Autodesk Inventor part; units mm, degrees
ref_plane "YZ Plane" through (0, 0, 0) normal (1, 0, 0) x (0, 1, 0)
ref_plane "XZ Plane" through (0, 0, 0) normal (0, 1, 0) x (-1, 0, 0)
ref_plane "XY Plane" through (0, 0, 0) normal (0, 0, 1) x (1, 0, 0)
sketch "Sketch1" plane through (0, 0, 0) normal (0, 1, 0) x (-1, 0, 0)
  line L0 (-15, 20.25) -> (15, 20.25)
  line L1 (15, 20.25) -> (15, -20.25)
  line L2 (15, -20.25) -> (-15, -20.25)
  line L3 (-15, -20.25) -> (-15, 20.25)
  line L4 (-15, 20.25) -> (15, -20.25) construction
  line L5 (15, 20.25) -> (-15, -20.25) construction
  point P0 (0, 0)
  dimension "d0" = 40.5
  dimension "d1" = 30
extrude "Plate1" add sketch "Sketch1" along normal blind 1.5
sketch "Sketch2" plane through (-15, 0, -21.75) normal (0, 0, 1) x (1, 0, 0)
  line L0 (30, 0) -> (0, 0)
  line L1 (0, 0) -> (0, 33.4)
  line L2 (0, 33.4) -> (30, 33.4)
  line L3 (30, 33.4) -> (30, 0)
edge flange "Flange1" height 33.4 angle 90 thickness 1.5 bend radius 0.31 thickness toward (0, 0, 1) relief tear relief width 1.5 relief depth 0.75 corner gap 0.31 corner form 0 edges at (0, 1.5, -20.25) (0, 1.5, 20.25) wall of the first edge with corners at (15, 0, -21.75) (-15, 0, -21.75) (-15, 33.4, -21.75) (15, 33.4, -21.75)
bend "Bend1"
corner "Corner1"
sketch "Sketch3" plane through (0, 1.5, 0) normal (0, 1, 0) x (1, 0, 0)
  circle A0 centre (7, 0) radius 0.7835
  circle A1 centre (0, -7) radius 0.7835
  circle A2 centre (-7, 0) radius 0.7835
  circle A3 centre (0, 7) radius 0.7835
  point P0 (0, 0)
hole "Hole1" at (0, 1.5, 7) at (7, 1.5, 0) at (-7, 1.5, 0) at (0, 1.5, -7) direction (0, -1, 0) diameter 2.1 depth 1.5
sketch "Sketch26" plane through (-15, 33.4, 21.75) normal (0, 0, 1) x (1, 0, 0)
  line L0 (30, 11.6) -> (25, 11.6)
  line L1 (25, 11.6) -> (25, -23.4)
  line L2 (25, -23.4) -> (30, -23.4)
  line L3 (30, -23.4) -> (30, 11.6)
  line L4 (0, 11.6) -> (5, 11.6)
  line L5 (5, 11.6) -> (5, -23.4)
  line L6 (5, -23.4) -> (0, -23.4)
  line L7 (0, -23.4) -> (0, 11.6)
  point P0 (15, -33.4)
  dimension "d91" = 35
  dimension "d92" = 5
  dimension "d93" = 10
  dimension "d94" = 10
  dimension "d95" = 5
  dimension "d96" = 35
  dimension "d97" = 10
  dimension "d98" = 10
extrude "Cut11" cut sketch "Sketch26" against normal blind 1.5
fillet "Corner Round1" radius 5 1 edges at (-15, 10, 21)
fillet "Corner Round2" radius 5 1 edges at (15, 10, 21)
mirror "Mirror1" about plane through (0, 0, 0) normal (0, 0, 1) of "Cut11"
fillet "Corner Round3" radius 5 1 edges at (-15, 10, -21)
fillet "Corner Round4" radius 5 1 edges at (15, 10, -21)
sketch "Sketch27" plane through (-15, 1.81, 21.75) normal (0, 0, 1) x (1, 0, 0)
  circle A0 centre (15, 32.29) radius 6
  point P0 (15, -1.81)
extrude "Cut12" cut sketch "Sketch27" against normal blind 1.5
sketch "Sketch28" plane through (15, 1.81, -21.75) normal (0, 0, -1) x (-1, 0, 0)
  circle A0 centre (15, 32.29) radius 6
  point P0 (15, -1.81)
extrude "Cut13" cut sketch "Sketch28" against normal blind 1.5
fillet "Corner Round5" radius 1 4 edges at (10, 33.4, -21) (10, 33.4, 21) (-10, 33.4, 21) (-10, 33.4, -21)
sketch "Sketch31" plane through (-15, 1.81, 21.75) normal (0, 0, 1) x (1, 0, 0)
  point P0 (15, -1.81)
sketch "Sketch32" plane through (-15, 1.81, 21.75) normal (0, 0, 1) x (1, 0, 0)
  circle A0 centre (23, 25.39) radius 0.7835
  circle A1 centre (22, 12.17) radius 0.7835
  circle A2 centre (7, 25.39) radius 0.7835
  circle A3 centre (8, 12.17) radius 0.7835
  circle A4 centre (15, 4.87) radius 0.7835
  point P0 (15, -1.81)
hole "Hole11" at (8, 27.2, 21.75) at (7, 13.98, 21.75) at (-8, 27.2, 21.75) at (-7, 13.98, 21.75) at (0, 6.68, 21.75) direction (0, 0, -1) diameter 2.1 depth 1.5
sketch "Sketch33" plane through (15, 1.81, -21.75) normal (0, 0, -1) x (-1, 0, 0)
  circle A0 centre (23.07, 4.19) radius 0.7835
  circle A1 centre (7.475, 4.69) radius 0.7835
  circle A2 centre (7.475, 19.79) radius 0.7835
  circle A3 centre (22.525, 19.79) radius 0.7835
  point P0 (15, -1.81)
hole "Hole12" at (7.525, 6.5, -21.75) at (-8.07, 6, -21.75) at (7.525, 21.6, -21.75) at (-7.525, 21.6, -21.75) direction (0, 0, 1) diameter 2.1 depth 1.5
sketch "Sketch34" plane through (0, 1.5, 0) normal (0, 1, 0) x (1, 0, 0)
  circle A0 centre (0, 0) radius 1.2295
  point P0 (0, 0)
hole "Hole13" at (0, 1.5, 0) direction (0, -1, 0) diameter 5.2 depth 1.5
equation "\"d18\" = Thickness"
equation "\"d99\" = Thickness"
equation "\"d105\" = Thickness"
equation "\"d107\" = Thickness"
equation "\"d129\" = Thickness"
equation "\"d136\" = Thickness"
equation "\"d143\" = Thickness"
equation "\"d2\" = Thickness"
equation "\"d3\" = BendReliefWidth"
equation "\"d4\" = BendReliefDepth"
equation "\"d5\" = MinimumRemnant"
equation "\"d6\" = TransitionRadius"
equation "\"d9\" = BendRadius"
equation "\"d10\" = CornerReliefSize"
equation "\"d11\" = GapSize"
equation "\"d12\" = JacobiRadiusSize"
equation "\"BendReliefWidth\" = Thickness"
equation "\"BendReliefDepth\" = 0.5 * Thickness"
equation "\"CornerReliefSize\" = 4 * Thickness"
equation "\"MinimumRemnant\" = 2 * Thickness"
equation "\"TransitionRadius\" = BendRadius"
equation "\"JacobiRadiusSize\" = BendRadius"
equation "\"GapSize\" = Thickness"
properties part number "axis_19_top_frame" material "Aluminum 6061-AHC"
Check sheet for the modelled part. Datum: model origin and axes. Units: mm. A direction names the side the tool comes from. Give positions to 0.01 mm unless a question says otherwise; leave off trailing zeros. Write each loop counter-clockwise with the first axis right and the second up, starting at its lowest first coordinate (ties: lowest second). Pieces come first, ordered by that corner, then holes.
Item 1: Cross-section at D-D (y = 6.5). Enter the section's corners in (x, z) (3 decimals).
Item 2: Access from +Z, -Z, +X, -X, +Y, -Y to the whole of each face (thin tool, end or side, straight path). Record for faces 1 (the face through (0, 14, 20.25)), 2 (the face through (-10, 21, 21)), 3 (the face through (-0.32, 5.68, 20.99)), 4 (the face through (10, 21, -21)).
Item 3: Draft check along Z on faces 5 (the face through (-7.05, 0.74, -1.05)), 6 (the face through (-7.57, 20.55, -20.99)), 7 (the face through (-0.21, 0.54, -21.23)). Enter one of: released by +Z, released by -Z, zero draft, split by the parting line, or undercut.
Item 4: Cross-section at A-A (y = 27.2). Enter the section's corners in (x, z), and give its area (3 significant figures).
Item 5: Cross-section at C-C (z = -0.5). Enter the section's corners in (x, y).
Item 6: Cross-section at B-B (z = -7). Enter the section's corners in (x, y).
Item 7: Scan lines: L1, parallel to X at y = 0.4, z = 0; L2, parallel to Z at x = 1.5, y = 8; L3, parallel to X at y = 6, z = -21.05. Record each from-to range of solid material in increasing order.
Item 8: Gauge pin test, flat ends, axial feed: pin 1 (3.5 mm diameter, centred on x = 7.525, y = 6.5, fed in from -Z); pin 2 (2.5 mm diameter, centred on x = 0, z = -7, fed in from +Y); pin 3 (1.6 mm diameter, centred on y = 25.5, z = 21, fed in from -X); pin 4 (0.8 mm diameter, centred on y = 26.5, z = 21, fed in from +X). Record the tip position at first contact, or that the pin passes through.
Report:
1. outline: (-14.77, -21.75) - (-8.993, -21.75) - (-8.993, -20.25) - (-14.77, -20.25) - close; (-14.77, 20.25) - (-1.034, 20.25) - (-1.034, 21.75) - (-14.77, 21.75) - close; (-7.147, -21.75) - (6.475, -21.75) - (6.475, -20.25) - (-7.147, -20.25) - close; (1.034, 20.25) - (14.77, 20.25) - (14.77, 21.75) - (1.034, 21.75) - close; (8.575, -21.75) - (14.77, -21.75) - (14.77, -20.25) - (8.575, -20.25) - close
2. face 1: +X, -X, +Y
2. face 2: +Z, -Z, -X, +Y
2. face 3: +Z
2. face 4: +Z, -Z, +X, +Y
3. face 5: undercut
3. face 6: zero draft
3. face 7: released by -Z
4. outline: (-10, -21.75) - (10, -21.75) - (10, -20.25) - (-10, -20.25) - close; (-10, 20.25) - (-9.05, 20.25) - (-9.05, 21.75) - (-10, 21.75) - close; (-6.95, 20.25) - (6.95, 20.25) - (6.95, 21.75) - (-6.95, 21.75) - close; (9.05, 20.25) - (10, 20.25) - (10, 21.75) - (9.05, 21.75) - close
4. area: 53.7 mm2
5. outline: (-15, 0) - (-7.92, 0) - (-7.92, 1.5) - (-15, 1.5) - close; (-6.08, 0) - (-2.55, 0) - (-2.55, 1.5) - (-6.08, 1.5) - close; (2.55, 0) - (6.08, 0) - (6.08, 1.5) - (2.55, 1.5) - close; (7.92, 0) - (15, 0) - (15, 1.5) - (7.92, 1.5) - close
6. outline: (-15, 0) - (-1.05, 0) - (-1.05, 1.5) - (-15, 1.5) - close; (1.05, 0) - (15, 0) - (15, 1.5) - (1.05, 1.5) - close
7. L1: x = -15 to -8.05, -5.95 to -2.6, 2.6 to 5.95, 8.05 to 15
7. L2: z = -21.75 to -20.25, 20.25 to 21.75
7. L3: x = -14.9 to -9.12, -7.02 to 6.6, 8.45 to 14.9
8. pin 1: stops at z = -21.75
8. pin 2: stops at y = 1.5
8. pin 3: stops at x = -10
8. pin 4: stops at x = 10
